The model under review builds one solid part; all positions refer to its coordinate system, in mm. A direction names the side the tool comes from. Give positions to 0.01 mm unless a question says otherwise; leave off trailing zeros. Loops run counter-clockwise (first coordinate to the right, second up) from the corner with the lowest first, then second, coordinate; pieces in that order, holes last. Notation, with made-up numbers: (47.5, -14.5) - (103.5, -14.5) arc R25 ccw to (103.5, 9.5) - close; hole circle Ø1 at (-19, 16). An arc over 180 degrees is marked (long way). Answer as a JSON object with one key per item and string values.
Autodesk Inventor part; units mm, degrees
ref_plane "YZ Plane" through (0, 0, 0) normal (1, 0, 0) x (0, 1, 0)
ref_plane "XZ Plane" through (0, 0, 0) normal (0, 1, 0) x (-1, 0, 0)
ref_plane "XY Plane" through (0, 0, 0) normal (0, 0, 1) x (1, 0, 0)
sketch "Sketch1" plane through (0, 0, 0) normal (0, 1, 0) x (-1, 0, 0)
  line L0 (0, 0) -> (60, 0)
  line L1 (60, 0) -> (60, -81)
  line L2 (60, -81) -> (0, -81)
  line L3 (0, -81) -> (0, 0)
  line L4 (45, -21.6284) -> (15, -21.6284) construction
  line L5 (45, -81) -> (45, 0) construction
  line L6 (15, 0) -> (15, -81) construction
  circle A0 centre (40, -73.5) radius 1.5
  circle A1 centre (40, -7.5) radius 1.5
  circle A2 centre (20, -7.5) radius 1.5
  circle A3 centre (20, -73.5) radius 1.5
  line L7 (60, -40.5) -> (0, -40.5) construction
  line L8 (30, 0) -> (30, -81) construction
  circle A4 centre (30, -40.5) radius 24
  circle A5 centre (30, -40.5) radius 27.5
  circle A6 centre (57.1293, -36) radius 1.5
  circle A7 centre (57.1293, -45) radius 1.5
  circle A8 centre (25.5, -13.3707) radius 1.5
  circle A9 centre (34.5, -13.3707) radius 1.5
  circle A10 centre (2.8707, -45) radius 1.5
  circle A11 centre (2.8707, -36) radius 1.5
  circle A12 centre (34.5, -67.6293) radius 1.5
  circle A13 centre (25.5, -67.6293) radius 1.5
  circle A14 centre (30, -40.5) radius 40 construction
  arc A15 (60, -81) -> (60, 0) centre (-17.0125, -40.5) ccw
  circle A16 centre (30, -40.5) radius 36.28 construction
  circle A17 centre (65.9998, -36) radius 1.5
  circle A18 centre (65.9998, -45) radius 1.5
  circle A19 centre (-5.9998, -45) radius 1.5
  circle A20 centre (-5.9998, -36) radius 1.5
  arc A21 (0, 0) -> (0, -81) centre (77.0125, -40.5) ccw
  line L9 (30, -40.5) -> (-3.3536, -73.8536) construction
  circle A22 centre (1.7157, -68.7843) radius 1.5
  circle A23 centre (11.8404, -76.1403) radius 1.5
  circle A24 centre (23.7426, -80.0075) radius 1.5
  circle A25 centre (36.2574, -80.0075) radius 1.5
  circle A26 centre (48.1596, -76.1403) radius 1.5
  circle A27 centre (58.2843, -68.7843) radius 1.5
  circle A28 centre (65.6403, -58.6596) radius 1.5
  circle A29 centre (69.5075, -46.7574) radius 1.5
  circle A30 centre (69.5075, -34.2426) radius 1.5
  circle A31 centre (65.6403, -22.3404) radius 1.5
  circle A32 centre (58.2843, -12.2157) radius 1.5
  circle A33 centre (48.1596, -4.8597) radius 1.5
  circle A34 centre (36.2574, -0.9925) radius 1.5
  circle A35 centre (23.7426, -0.9925) radius 1.5
  circle A36 centre (11.8404, -4.8597) radius 1.5
  circle A37 centre (1.7157, -12.2157) radius 1.5
  circle A38 centre (-5.6403, -22.3404) radius 1.5
  circle A39 centre (-9.5075, -34.2426) radius 1.5
  circle A40 centre (-9.5075, -46.7574) radius 1.5
  circle A41 centre (-5.6403, -58.6596) radius 1.5
  circle A42 centre (48.1596, -68.7843) radius 1.5
  circle A43 centre (48.1596, -12.2157) radius 1.5
  circle A44 centre (11.8404, -12.2157) radius 1.5
  circle A45 centre (11.8404, -68.7843) radius 1.5
  line L10 (0, 0) -> (6, 0)
  arc A46 (6, 0) -> (6.3936, -12.9505) centre (40.8143, -5.423) ccw
  arc A47 (6.3936, -12.9505) -> (-5.0141, -31) centre (30, -40.5) ccw
  line L11 (-9.4798, -31) -> (7.9603, -31)
  line L12 (-10, -40.5) -> (70, -40.5) construction
  line L13 (-18.775, -8.5) -> (-32.775, -8.5)
  line L14 (-32.775, -8.5) -> (-32.775, -26.5)
  line L15 (-32.775, -26.5) -> (-18.775, -26.5)
  line L16 (-18.775, -26.5) -> (-18.775, -8.5)
  line L17 (-18.775, -54.5) -> (-37.775, -54.5)
  line L18 (-37.775, -54.5) -> (-37.775, -68.5)
  line L19 (-37.775, -68.5) -> (-18.775, -68.5)
  line L20 (-18.775, -68.5) -> (-18.775, -54.5)
  line L21 (-17.0125, -40.5) -> (-69.0232, -40.5)
  line L22 (-16.775, -6.5) -> (-23.775, -6.5)
  line L23 (-23.775, -6.5) -> (-23.775, -28.5)
  line L24 (-23.775, -28.5) -> (-16.775, -28.5)
  line L25 (-16.775, -28.5) -> (-16.775, -6.5)
  line L26 (-16.775, -52.5) -> (-23.775, -52.5)
  line L27 (-23.775, -52.5) -> (-23.775, -70.5)
  line L28 (-23.775, -70.5) -> (-16.775, -70.5)
  line L29 (-16.775, -70.5) -> (-16.775, -52.5)
  circle A48 centre (-30.7674, -10.5) radius 1.25
  circle A49 centre (-30.7674, -24.5) radius 1.25
  circle A50 centre (-35.775, -56.5) radius 1.25
  line L30 (-16.775, -32.5) -> (-49.775, -32.5)
  line L31 (-51.775, -34.5) -> (-51.775, -46.5)
  line L32 (-49.775, -48.5) -> (-16.775, -48.5)
  line L33 (-16.775, -48.5) -> (-16.775, -32.5)
  line L34 (-16.775, -43.5) -> (-38.775, -43.5) construction
  line L35 (-32.0174, -32.5) -> (-46.0174, -32.5)
  line L36 (-46.0174, -32.5) -> (-46.0174, -48.5)
  line L37 (-46.0174, -48.5) -> (-32.0174, -48.5)
  line L38 (-32.0174, -48.5) -> (-32.0174, -32.5)
  line L39 (0, 0) -> (-59.1614, -10.4318)
  line L40 (0, -81) -> (-59.1614, -70.5682)
  arc A51 (-51.775, -9.1293) -> (-51.775, -71.8707) centre (29.3856, -40.5) ccw
  arc A52 (-49.775, -32.5) -> (-51.775, -34.5) centre (-49.775, -34.5) ccw
  arc A53 (-51.775, -46.5) -> (-49.775, -48.5) centre (-49.775, -46.5) ccw
  arc A54 (6.3936, -68.0495) -> (6, -81) centre (40.8143, -75.577) ccw
  arc A55 (-5.0141, -50) -> (6.3936, -68.0495) centre (30, -40.5) ccw
  line L41 (-9.4798, -50) -> (7.9603, -50)
  arc A56 (-4.4033, -0.7764) -> (-4.4033, -80.2236) centre (73.0125, -40.5) ccw
  circle A57 centre (1.7157, -12.2157) radius 3.25
  circle A58 centre (1.7157, -68.7843) radius 3.25
  arc A59 (6.3936, -12.9505) -> (7.0417, -15.4657) centre (40.8143, -5.423) ccw
  arc A60 (7.0417, -15.4657) -> (0, -20.0981) centre (14.8139, -34.9486) ccw
  arc A61 (7.0417, -65.5343) -> (6.3936, -68.0495) centre (40.8143, -75.577) ccw
  arc A62 (0, -60.9019) -> (7.0417, -65.5343) centre (14.8139, -46.0514) ccw
  point P0 (30, -21.6284)
  point P1 (-18.775, -17.5)
  point P2 (-18.775, -61.5)
  point P3 (-51.775, -48.5)
  point P4 (-51.775, -32.5)
  point P5 (-16.775, -40.5)
  point P6 (-16.775, -61.5)
  point P7 (-51.775, -40.5)
  point P8 (-14, -40.5)
  point P9 (6, -81)
  point P10 (0, -60.9019)
  dimension "d18" = 48
  dimension "d6" = 60
  dimension "d7" = 81
  dimension "d8" = 3
  dimension "d9" = 7.5
  dimension "d10" = 5
  dimension "d11" = 30
  dimension "d12" = 3
  dimension "d13" = 7.5
  dimension "d14" = 5
  dimension "d15" = 3
  dimension "d16" = 3
  dimension "d17" = 5
  dimension "d19" = 55
  dimension "d20" = 3
  dimension "d21" = 4.5
  dimension "d22" = 3
  dimension "d23" = 4.5
  dimension "d24" = 360
  dimension "d25" = 80
  dimension "d26" = 72.56
  dimension "d27" = 3
  dimension "d28" = 3
  dimension "d29" = 360
  dimension "d30" = 45
  dimension "d31" = 3
  dimension "d32" = 360
  dimension "d33" = 3
  dimension "d34" = 3
  dimension "d35" = 3
  dimension "d36" = 3
  dimension "d37" = 6
  dimension "d38" = 5
  dimension "d39" = 30
  dimension "d40" = 40.5
  dimension "d41" = 14
  dimension "d42" = 18
  dimension "d43" = 19
  dimension "d44" = 14
  dimension "d45" = 7
  dimension "d46" = 2
  dimension "d47" = 2
  dimension "d48" = 2
  dimension "d49" = 2
  dimension "d50" = 2
  dimension "d51" = 2
  dimension "d52" = 7
  dimension "d53" = 2.5
  dimension "d54" = 2.5
  dimension "d55" = 2
  dimension "d56" = 2
  dimension "d57" = 2.5
  dimension "d58" = 2
  dimension "d59" = 2
  dimension "d60" = 35
  dimension "d61" = 16
  dimension "d62" = 4
  dimension "d63" = 4
  dimension "d64" = 22
  dimension "d65" = 14
  dimension "d66" = 80
  dimension "d67" = 80
  dimension "d68" = 2
  dimension "d69" = 4
  dimension "d78" = 6.5
extrude "Extrusion1" add sketch "Sketch1" along normal blind 2 contours L0 A46 A47 L3 A57 | L3 A57 A47 L11 A21 | A21 A39 A40 L40 A56 L39 | A59 A60 A47 | A21 A39 | L3 A58 A55 A54 L2 | A21 L41 A55 L3 A58 | A21 A40 | A62 A61 A55 picked at (-10.1825, -34.1938) picked at (-10.1825, -46.8062)
extrude "Extrusion2" add sketch "Sketch1" against normal blind 4 contours A21 A39 A40 L40 A56 L39 | A21 A39 | A21 A40 picked at (-10.1825, -34.1938) picked at (-10.1825, -46.8062)
ref_plane "Work Plane1" through (0, -5.5, 0) normal (0, -1, 0) x (1, 0, 0)
sketch "Sketch2" plane through (0, -5.5, 0) normal (0, -1, 0) x (1, 0, 0)
  line L0 (0, -81) -> (59.1614, -70.5682)
  arc A0 (51.775, -71.8707) -> (51.775, -9.1293) centre (-29.3856, -40.5) ccw
  line L1 (49.775, -48.5) -> (16.775, -48.5)
  arc A1 (49.775, -48.5) -> (51.775, -46.5) centre (49.775, -46.5) ccw
  line L2 (51.775, -34.5) -> (51.775, -46.5)
  arc A2 (51.775, -34.5) -> (49.775, -32.5) centre (49.775, -34.5) ccw
  line L3 (16.775, -32.5) -> (49.775, -32.5)
  line L4 (46.0174, -32.5) -> (46.0174, -48.5)
  line L5 (32.0174, -48.5) -> (32.0174, -32.5)
  line L6 (16.775, -48.5) -> (16.775, -32.5)
  arc A3 (4.4033, -80.2236) -> (4.4033, -0.7764) centre (-73.0125, -40.5) ccw
  arc A4 (0, -81) -> (0, 0) centre (-77.0125, -40.5) ccw
  line L7 (37.775, -68.5) -> (18.775, -68.5)
  line L8 (37.775, -54.5) -> (37.775, -68.5)
  line L9 (18.775, -54.5) -> (37.775, -54.5)
  circle A5 centre (35.775, -56.5) radius 1.25
  line L10 (23.775, -52.5) -> (23.775, -70.5)
  line L11 (23.775, -70.5) -> (16.775, -70.5)
  line L12 (16.775, -70.5) -> (16.775, -52.5)
  line L13 (18.775, -68.5) -> (18.775, -54.5)
  line L14 (16.775, -52.5) -> (23.775, -52.5)
  line L15 (32.775, -26.5) -> (18.775, -26.5)
  circle A6 centre (30.7674, -24.5) radius 1.25
  line L16 (32.775, -8.5) -> (32.775, -26.5)
  circle A7 centre (30.7674, -10.5) radius 1.25
  line L17 (18.775, -8.5) -> (32.775, -8.5)
  line L18 (0, 0) -> (59.1614, -10.4318)
  line L19 (23.775, -6.5) -> (23.775, -28.5)
  line L20 (16.775, -6.5) -> (23.775, -6.5)
  line L21 (16.775, -28.5) -> (16.775, -6.5)
  line L22 (18.775, -26.5) -> (18.775, -8.5)
  line L23 (23.775, -28.5) -> (16.775, -28.5)
  line L24 (17.0125, -40.5) -> (69.0232, -40.5)
  point P0 (23.775, -26.5)
  point P1 (23.775, -8.5)
  point P2 (23.775, -68.5)
  point P3 (23.775, -54.5)
extrude "Extrusion3" add sketch "Sketch2" along normal blind 2.5 contours A4 L18 A3 L0 | L2 A1 L1 L4 L24 | L24 L4 L3 A2 L2 | A3 L18 A0 L0 | L5 L1 L6 L3 | L7 L10 L9 L8 | L15 L19 L17 L16
extrude "Extrusion4" add sketch "Sketch2" against normal up to surface (1.5 mm away) contours A4 L18 A3 L0
fillet "Fillet1" radius 2 3 edges at (46.0174, -6.75, -32.5) (46.0174, -6.75, -48.5) (14, -5.5, -40.5)
fillet "Fillet2" radius 15 2 edges at (0, 1, -20.0981) (0, 1, -60.9019)
equation "\"d11\" = 0.5 * d6"
equation "\"d12\" = d8"
equation "\"d15\" = d8"
equation "\"d16\" = d8"
equation "\"d22\" = d8"
equation "\"d27\" = d8"
equation "\"d28\" = d8"
equation "\"d31\" = d8"
equation "\"d33\" = d8"
equation "\"d34\" = d8"
equation "\"d35\" = d8"
equation "\"d36\" = d8"
properties part number "SensorHolder"
Q1. Consider section A-A, the plane x = 40.5. State the section outline as (y, z) points.
Results:
{"outline": "(-8, -73.86) - (-5.5, -73.86) - (-5.5, -48.5) - (-8, -48.5) - close; (-8, -32.5) - (-5.5, -32.5) - (-5.5, -7.14) - (-8, -7.14) - close"}
Q2. For faces 1 (the face through (57.626, -6.732, -40.051)), 2 (the face through (1, 0, -65)), 3 (the face through (23.775, -7, -61)), 4 (the face through (-5.1, 0.986, -64.642)), 5 (the face through (14, -1, -41)), list the 3-axis set-ups (+Z, -Z, +X, -X, +Y, -Y) from which the entire face can be reached by the end or side of a thin tool; tool diameter is ignored.
Results:
{"face 1": "+X, +Y, -Y", "face 2": "-X, -Y", "face 3": "+Y, -Y", "face 4": "-X, +Y, -Y", "face 5": "+X, +Y"}
Q3. Consider section D-D, the plane y = -1.5. State the section outline as (x, z) points (1 decimal).
Results:
{"outline": "(0, -81) - (4.4, -80.2) arc R87 ccw to (4.4, -0.8) - (0, 0) arc R87 cw to start"}
Q4. Clearance check with flat-ended pins moving along their axes: pin 1 Ø5 at (x, z) = (5.64, -22.34) entering from +Y; pin 2 Ø0.8 at (x, y) = (19, -6.5) entering from -Z; pin 3 Ø1.5 at (x, z) = (43, -13) entering from +Y; pin 4 Ø1.6 at (x, y) = (7.5, 1.5) entering from -Z. State where each tip first meets the part, or that it passes through.
Results:
{"pin 1": "stops at y = 2", "pin 2": "stops at z = -77.72", "pin 3": "stops at y = -5.5", "pin 4": "stops at z = -75.39"}
Q5. To check wall thickness, follow probe 1 along Z at (x, y) = (17, -6); probe 2 along Y at (x, z) = (8, -23); probe 3 along X at (y, z) = (-7, -39.5). State the ranges of each line that lie inside material, in increasing order. Write a range as [from, to].
Results:
{"probe 1": "z = [-78, -70.5], [-52.5, -28.5], [-6.5, -3]", "probe 2": "y = [0, 2]", "probe 3": "x = [9.99, 32.02], [46.02, 57.62]"}
Q6. Consider section B-B, the plane y = -6.5. State how many separate pieces and enclosed holes the cut face has, plus the area to 3 significant figures.
Results:
{"separate pieces": "1", "enclosed holes": "6", "area": "2,900 mm^2"}
